Geometry check sheet. Reference: the model listing, model coordinates, mm. A direction names the side the tool comes from. Round coordinates to 2 decimals unless told otherwise and drop trailing zeros. Order: outer loops, then holes, each group sorted by start corner. A loop starts at its lowest first (then second) coordinate and runs counter-clockwise, first axis right, second up.
(1) Cross-section at C-C on x = 5.25. Enter the section's corners in (y, z), and give its area (3 significant figures).
(2) Set-up check for faces 1 (the face through (9.307, -2.438, 0.108)), 2 (the face through (8.8, 0, 0)), 3 (the face through (7.68, 1.917, -2.5)): record each of +Z, -Z, +X, -X, +Y, -Y from which the full face is reachable in a straight line by a thin tool's end or side.
(3) Draft check along Z on faces 4 (the face through (2.7, -3.7, -0.4)), 5 (the face through (2.7, 3.7, 0.4)), 6 (the face through (9.8, 0, 0)), 7 (the face through (6.8, -0.1, -2.5)). Enter one of: pulls with the +Z half, pulls with the -Z half, needs draft (parallel to the pull), parting line crosses it, or undercut.
(4) Gauge pin test, flat ends, axial feed: P1, Ø1.5, axis at x = 1, z = 1.5, coming from the -Y side; P2, Ø3, axis at y = 0, z = 0, coming from the -X side; P3, Ø4, axis at x = 3.5, y = -2.5, coming from the +Z side. Record the tip position at first contact, or that the pin passes through.
(5) Thickness scan on L1, parallel to Y at x = 9.1, z = 0; L2, parallel to Y at x = 2, z = 0; L3, parallel to X at y = 0, z = 0.25. Record the ranges inside material, lowest first.
(6) Cross-section at A-A on x = 1.5. Enter the section's corners in (y, z).
(7) Cross-section at B-B on z = 0. Enter the section's corners in (x, y).
from build123d import *

# Parameters (mm, degrees)
SKETCH2_W           = 0.8
SKETCH2_H           = 1
BOSS_EXTRUDE1_DEPTH = 5.5
CHAMFER1_SIZE       = 0.5
FILLET1_SIZE        = 0.5
FILLET1_SIZE_2      = 0.8
SKETCH3_R           = 0.5
CUT_EXTRUDE1_DEPTH  = 10


with BuildPart() as part:
    # Sketch1 → Revolve1 (revolve)
    with BuildSketch(Plane.XY, mode=Mode.PRIVATE) as revolve1_sk:
        Polygon((8.8, 0), (8.8, 2.5), (4.85, 2.5), (4.85, 2.75), (0, 2.75), (0, 3.4), (5.5, 3.4), (5.5, 3.15), (9.8, 3.15), (9.8, 0), align=None)
    revolve(revolve1_sk.sketch.rotate(Axis((0, 0, 0), (1, 0, 0)), 90), axis=Axis((0, 0, 0), (1, 0, 0)))

    # Sketch2 → Boss-Extrude1 (add)
    with BuildSketch(Plane.ZY):
        with Locations((0, 3.45)):
            Rectangle(SKETCH2_W, SKETCH2_H)
        with Locations((0, -3.45)):
            Rectangle(SKETCH2_W, SKETCH2_H)
    extrude(amount=-BOSS_EXTRUDE1_DEPTH)

    # Chamfer1
    chamfer1_edges = [part.edges().sort_by_distance(p)[0] for p in [
        (0, 3.95, 0),
        (0, -3.95, 0),
    ]]
    chamfer(chamfer1_edges, length=CHAMFER1_SIZE)

    # Fillet1
    # an asymmetric fillet: 0.8, 0.5 mm, written as the material it takes off along each edge
    with BuildSketch(Plane(origin=(0, 0, 0), x_dir=(0, -0.8910585432976912, -0.45388839202627373), z_dir=(0, 0.45388839202627373, -0.8910585432976912))) as fillet1_piece_1_section:
        with BuildLine():
            Bezier((3.4 - FILLET1_SIZE, 0), (3.4, 0), (3.4, -FILLET1_SIZE_2), weights=[1, 0.707106781, 1])
            Line((3.4, -FILLET1_SIZE_2), (3.4, 0))
            Line((3.4, 0), (3.4 - FILLET1_SIZE, 0))
        make_face()
    fillet1_piece_1 = revolve(axis=Axis((0, 0, 0), (-1, 0, 0)), revolution_arc=233.986868401, mode=Mode.PRIVATE)
    fillet1_piece_1 = split(fillet1_piece_1, bisect_by=Plane(origin=(0.182093779, -3.13232652, -0.4), z_dir=(0, 0, -1)), keep=Keep.TOP, mode=Mode.PRIVATE)
    add(fillet1_piece_1, mode=Mode.SUBTRACT)
    with BuildSketch(Plane(origin=(0, 0, 0), x_dir=(0, -0.8910585432976912, -0.45388839202627373), z_dir=(0, 0.45388839202627373, -0.8910585432976912))) as fillet1_piece_2_section:
        with BuildLine():
            Bezier((3.4 - FILLET1_SIZE, 0), (3.4, 0), (3.4, -FILLET1_SIZE_2), weights=[1, 0.707106781, 1])
            Line((3.4, -FILLET1_SIZE_2), (3.4, 0))
            Line((3.4, 0), (3.4 - FILLET1_SIZE, 0))
        make_face()
    fillet1_piece_2 = revolve(axis=Axis((0, 0, 0), (-1, 0, 0)), revolution_arc=233.986868401, mode=Mode.PRIVATE)
    fillet1_piece_2 = split(fillet1_piece_2, bisect_by=Plane(origin=(0.229357983, 0, 0.4), z_dir=(0, 0, 1)), keep=Keep.TOP, mode=Mode.PRIVATE)
    add(fillet1_piece_2, mode=Mode.SUBTRACT)
    with BuildSketch(Plane(origin=(0, 0, 0), x_dir=(0, -0.8910585432977036, 0.4538883920262497), z_dir=(0, 0.4538883920262497, 0.8910585432977036))) as fillet1_piece_3_section:
        with BuildLine():
            Bezier((3.4 - FILLET1_SIZE, 0), (3.4, 0), (3.4, FILLET1_SIZE_2), weights=[1, 0.707106781, 1])
            Line((3.4, FILLET1_SIZE_2), (3.4, 0))
            Line((3.4, 0), (3.4 - FILLET1_SIZE, 0))
        make_face()
    fillet1_piece_3 = revolve(axis=Axis((0, 0, 0), (1, 0, 0)), revolution_arc=233.986868401, mode=Mode.PRIVATE)
    fillet1_piece_3 = split(fillet1_piece_3, bisect_by=Plane(origin=(0.18209405, -3.132326501, 0.4), z_dir=(0, 0, 1)), keep=Keep.TOP, mode=Mode.PRIVATE)
    add(fillet1_piece_3, mode=Mode.SUBTRACT)
    with BuildSketch(Plane(origin=(0, 0, 0), x_dir=(0, -0.8910585432977036, 0.4538883920262497), z_dir=(0, 0.4538883920262497, 0.8910585432977036))) as fillet1_piece_4_section:
        with BuildLine():
            Bezier((3.4 - FILLET1_SIZE, 0), (3.4, 0), (3.4, FILLET1_SIZE_2), weights=[1, 0.707106781, 1])
            Line((3.4, FILLET1_SIZE_2), (3.4, 0))
            Line((3.4, 0), (3.4 - FILLET1_SIZE, 0))
        make_face()
    fillet1_piece_4 = revolve(axis=Axis((0, 0, 0), (1, 0, 0)), revolution_arc=233.986868401, mode=Mode.PRIVATE)
    fillet1_piece_4 = split(fillet1_piece_4, bisect_by=Plane(origin=(0.229357983, 0, -0.4), z_dir=(0, 0, -1)), keep=Keep.TOP, mode=Mode.PRIVATE)
    add(fillet1_piece_4, mode=Mode.SUBTRACT)

    # Sketch3 → Cut-Extrude1 (cut)
    with BuildSketch(Plane(origin=(9.8, 0, 0), x_dir=(0, 0, -1), z_dir=(1, 0, 0))):
        with Locations((0, -1.95)):
            Circle(SKETCH3_R)
    extrude(amount=-CUT_EXTRUDE1_DEPTH, mode=Mode.SUBTRACT)


solid = part.part
Found:
1. outline: (-3.95, -0.4) - (-3.38, -0.4) arc R3.4 ccw to (3.38, -0.4) - (3.95, -0.4) - (3.95, 0.4) - (3.38, 0.4) arc R3.4 ccw to (-3.38, 0.4) - (-3.95, 0.4) - close; hole circle Ø5 at (0, 0)
1. area: 17.6 mm2
2. face 1: +X, -X
2. face 2: -X
2. face 3: +X
3. face 4: pulls with the -Z half
3. face 5: pulls with the +Z half
3. face 6: needs draft
3. face 7: undercut
4. P1: stops at y = -3.32
4. P2: stops at x = 8.8
4. P3: stops at z = 3.36
5. L1: y = -3.15 to -2.45, -1.45 to 3.15
5. L2: y = -3.95 to -2.75, 2.75 to 3.95
5. L3: x = 8.8 to 9.8
6. outline: (-3.95, -0.4) - (-3.38, -0.4) arc R3.4 ccw to (3.38, -0.4) - (3.95, -0.4) - (3.95, 0.4) - (3.38, 0.4) arc R3.4 ccw to (-3.38, 0.4) - (-3.95, 0.4) - close; hole circle Ø5.5 at (0, 0)
7. outline: (0, -3.45) - (0.5, -3.95) - (5.5, -3.95) - (5.5, -3.15) - (9.8, -3.15) - (9.8, -2.45) - (8.8, -2.45) - (8.8, -2.5) - (4.85, -2.5) - (4.85, -2.75) - (0, -2.75) - close; (0, 2.75) - (4.85, 2.75) - (4.85, 2.5) - (8.8, 2.5) - (8.8, -1.45) - (9.8, -1.45) - (9.8, 3.15) - (5.5, 3.15) - (5.5, 3.95) - (0.5, 3.95) - (0, 3.45) - close
